The drawing under review shows one solid part. Ordinate dimensions are in mm from its lowest x, y, z. A direction names the side the tool comes from. Round coordinates to 2 decimals unless told otherwise and drop trailing zeros. Write each loop counter-clockwise with the first axis right and the second up, starting at its lowest first coordinate (ties: lowest second). Pieces come first, ordered by that corner, then holes. Notation, with made-up numbers: (83.5, 89.5) -> (93.5, 89.5) arc R20 cw to (93.5, 121.5) -> close; hole circle Ø5 at (2, -38). An arc over 180 degrees is marked (long way). Use CSV: the item, a comma, the result in double quotes. Start each with the question number.
1) Take a section at A-A, the plane x = 3.25. Give the boundary of the cut face in (y, z) (1 decimal).
2) Machinability: for the marked faces 4, 5 and 6, which of the approach directions +Z, -Z, +X, -X, +Y, -Y give a long, thin tool a straight path to every point of the face, cutting with its end or side? Answer none if there is none.
3) Wall thickness on probe 1 along Y at (x, z) = (2.2, 1.05) (1 decimal); probe 2 along Y at (x, z) = (2.55, 1.55) (1 decimal); probe 3 along Z at (x, y) = (1.85, 10) (1 decimal): over which ranges is each line inside the solid? List them lowest first. Write a range as [from, to].
4) Mouldability with a two-part tool opening along X and no side actions: class the marked faces 1, 2 and 3 as released by +X, released by -X, zero draft, split by the parting line, or undercut.
5) Take a section at D-D, the plane x = 0.45. Give the boundary of the cut face in (y, z) (1 decimal), then the cut area to 3 significant figures.
6) Take a section at B-B, the plane z = 3.1. Give the boundary of the cut face in (x, y) (1 decimal).
7) For pin 1 Ø2 at (x, y) = (2.5, 11) entering from +Z; pin 2 Ø1 at (y, z) = (16, 3) entering from -X; pin 3 Ø2 at (x, z) = (3.5, 3) entering from -Y; pin 4 Ø1 at (y, z) = (16, 4) entering from -X, all flat-tipped, find the tip position at first contact; note any pin that passes through.
8) Take a section at C-C, the plane y = 9.25. Give the boundary of the cut face in (x, z) (1 decimal).
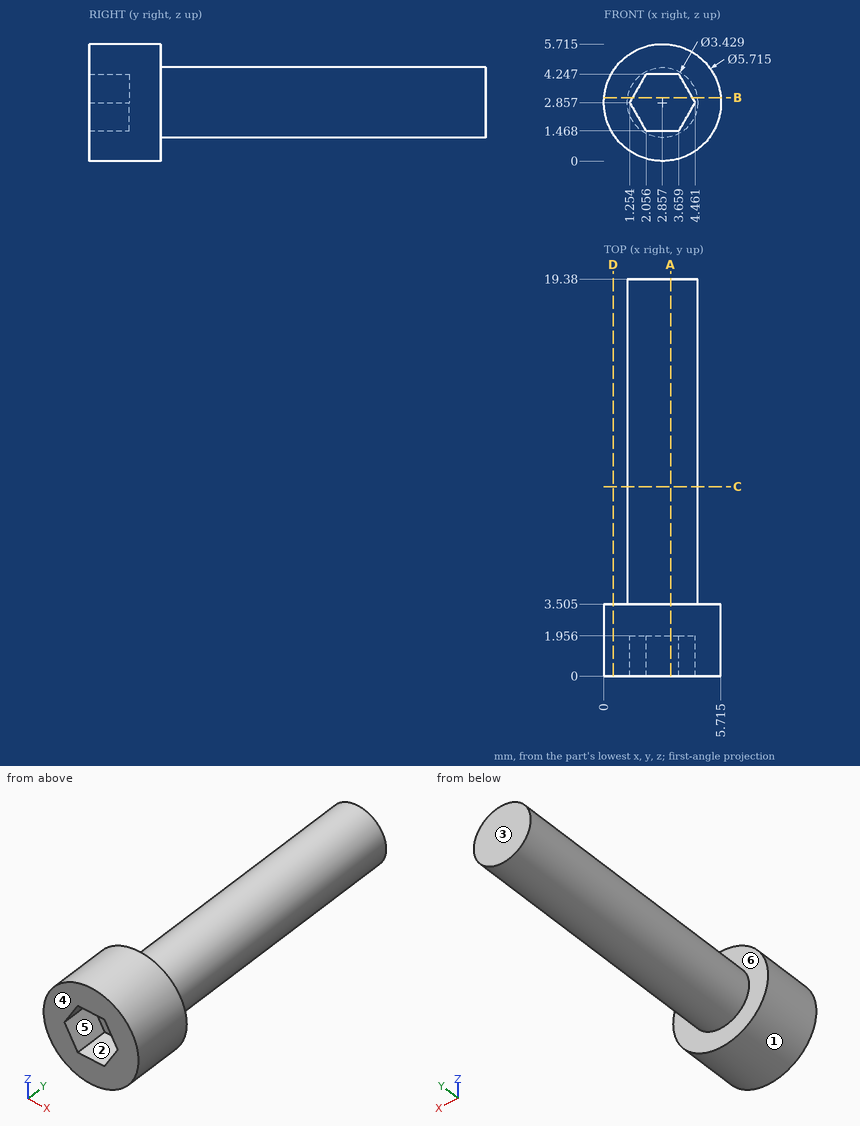
Values found:
1,outline,"(0, 0) -> (3.5, 0) -> (3.5, 1.2) -> (19.4, 1.2) -> (19.4, 4.5) -> (3.5, 4.5) -> (3.5, 5.7) -> (0, 5.7) -> (0, 4.2) -> (2, 4.2) -> (2, 1.5) -> (0, 1.5) -> close"
2,face 4,"+Z, -Z, +X, -X, -Y"
2,face 5,"-Y"
2,face 6,"+Y"
3,probe 1,"[0, 3.5]"
3,probe 2,"[2, 19.4]"
3,probe 3,"[1.5, 4.2]"
4,face 1,"split by the parting line"
4,face 2,"undercut"
4,face 3,"zero draft"
5,outline,"(0, 1.3) -> (3.5, 1.3) -> (3.5, 4.4) -> (0, 4.4) -> close"
5,area,"10.8 mm²"
6,outline,"(0, 0) -> (1.4, 0) -> (1.4, 2) -> (4.3, 2) -> (4.3, 0) -> (5.7, 0) -> (5.7, 3.5) -> (4.6, 3.5) -> (4.6, 19.4) -> (1.2, 19.4) -> (1.2, 3.5) -> (0, 3.5) -> close"
7,pin 1,"z = 4.57"
7,pin 2,"x = 1.14"
7,pin 3,"y = 0"
7,pin 4,"x = 1.27"
8,outline,"circle Ø3.4 at (2.9, 2.9)"
